For this review, take the finished solid that the model builds, in its own axes (mm). A direction names the side the tool comes from. Round coordinates to 2 decimals unless told otherwise and drop trailing zeros. Loops run counter-clockwise (first coordinate to the right, second up) from the corner with the lowest first, then second, coordinate; pieces in that order, holes last.
1) Wall thickness on L1, parallel to X at y = 3, z = -3; L2, parallel to Y at x = 3.75, z = 3.5; L3, parallel to Y at x = -1.75, z = 1.75: over which ranges is each line inside the solid? List them lowest first.
2) Take a section at B-B (z = 0). State the section outline as (x, y) points, then the cut area to 3 significant figures.
3) Tool access review of faces 1 (the flat face through (4.57, 0.49, -4.58)), 2 (the cylindrical face through (-1.08, 5.39, 4.88)): name each direction out of +Z, -Z, +X, -X, +Y, -Y from which nothing blocks a thin tool from reaching the whole face with its end or side.
4) Insertion check: pin 1 (1.5 mm diameter, centred on x = 3.5, y = 6.5, fed in from +Z); pin 2 (1 mm diameter, centred on x = -2, z = -2, fed in from -Y); pin 3 (3 mm diameter, centred on x = 1, y = 4.5, fed in from +Z); pin 4 (0.5 mm diameter, centred on x = 0, z = 5.5, fed in from +Y). Each pin has a flat end and moves straight along its axis. Give the tip position at first contact, or say it passes through.
5) Take a section at C-C (y = 5). State the section outline as (x, z) points, then the cut area to 3 significant figures.
```python
from build123d import *

# Parameters (mm, degrees)
BOSS_EXTRUDE1_DEPTH = 1
SKETCH3_R           = 5
BOSS_EXTRUDE2_DEPTH = 10.2
FILLET1_R           = 0.3
SKETCH4_W           = 0.9
SKETCH4_H           = 3.5
BOSS_EXTRUDE3_DEPTH = 0.3
BOSS_EXTRUDE4_DEPTH = 0.01


with BuildPart() as part:
    # Sketch2 → Boss-Extrude1 (new body)
    with BuildSketch(Plane(origin=(0, 0, 0), x_dir=(1, 0, 0), z_dir=(0, 1, 0))):
        Polygon((5.15, -5.15), (-5.15, -5.15), (-5.15, 4), (-4, 5.15), (4, 5.15), (5.15, 4), align=None)
    extrude(amount=BOSS_EXTRUDE1_DEPTH)

    # Sketch3 → Boss-Extrude2 (add)
    with BuildSketch(Plane(origin=(0, 0, 0), x_dir=(1, 0, 0), z_dir=(0, 1, 0))):
        Circle(SKETCH3_R)
    extrude(amount=BOSS_EXTRUDE2_DEPTH)

    # Fillet1
    fillet1_edges = [part.edges().sort_by_distance(p)[0] for p in [
        (-5, 10.2, 0),
    ]]
    fillet(fillet1_edges, radius=FILLET1_R)

    # Sketch4 → Boss-Extrude3 (add)
    with BuildSketch(Plane(origin=(0, 0, 0), x_dir=(1, 0, 0), z_dir=(0, 1, 0))):
        with Locations((0, 4.05)):
            Rectangle(SKETCH4_W, SKETCH4_H)
        with Locations((0, -4.05)):
            Rectangle(SKETCH4_W, SKETCH4_H)
    extrude(amount=BOSS_EXTRUDE3_DEPTH)

    # Sketch5 → Boss-Extrude4 (add)
    with BuildSketch(Plane(origin=(0, 10.2, 0), x_dir=(1, 0, 0), z_dir=(0, 1, 0))):
        with BuildLine():
            Line((-4.077855221, -2.336898969), (4.077855221, -2.336898969))
            ThreePointArc((4.077855221, -2.336898969), (0, -4.7), (-4.077855221, -2.336898969))
        make_face()
    extrude(amount=BOSS_EXTRUDE4_DEPTH)


solid = part.part
```
Response:
1. L1: x = -4 to 4
1. L2: y = 0 to 1
1. L3: y = 0 to 10.2
2. outline: (-5.15, 0) - (5.15, 0) - (5.15, 1) - (5, 1) - (5, 9.9) arc R0.3 ccw to (4.7, 10.2) - (-4.7, 10.2) arc R0.3 ccw to (-5, 9.9) - (-5, 1) - (-5.15, 1) - close
2. area: 102 mm2
3. face 1: -Z, +X, +Y, -Y
3. face 2: +Y
4. pin 1: stops at z = 4.18
4. pin 2: stops at y = 0
4. pin 3: stops at z = 5
4. pin 4: stops at y = 0.3
5. outline: circle Ø10 at (0, 0)
5. area: 78.5 mm2
